```python
from build123d import *

# Parameters (mm, degrees)
SKETCH1_R               = 21
SKETCH1_R_2             = 17
BOSS_EXTRUDE1_DEPTH     = 6
SKETCH2_W               = 42
SKETCH2_H               = 3
CUT_EXTRUDE1_DEPTH      = 25.812
SKETCH3_W               = 34
SKETCH3_H               = 6
SKETCH3_W_2             = 33.201655863
SKETCH3_H_2             = 2.84
BOSS_EXTRUDE2_DEPTH     = 5.334
CUT_EXTRUDE2_START      = -19.05
SKETCH4_R               = 24.04163056
SKETCH4_R_2             = 21
CUT_EXTRUDE2_DEPTH      = 19.05
SKETCH5_R               = 1.4
CUT_EXTRUDE3_DEPTH      = 19.05
CHAMFER1_SIZE           = 1.279400032
CHAMFER2_SIZE           = 1.279400032
FILLET2_R               = 1.27
SKETCH8_R               = 0.85
CUT_EXTRUDE7_DEPTH      = 15.494
FILLET3_R               = 1.27
CUT_EXTRUDE8_DEPTH      = 19.812
CUT_EXTRUDE8_DEPTH_BACK = 28.194
SKETCH9_R               = 0.875


with BuildPart() as part:
    # Sketch1 → Boss-Extrude1 (new body)
    with BuildSketch(Plane(origin=(0, 0, 0), x_dir=(1, 0, 0), z_dir=(0, 1, 0))):
        with Locations(Location((0, 0, 0), (0, 0, 270))):
            Circle(SKETCH1_R)
        with Locations(Location((0, 0, 0), (0, 0, 270))):
            Circle(SKETCH1_R_2, mode=Mode.SUBTRACT)
    extrude(amount=BOSS_EXTRUDE1_DEPTH)

    # Sketch2 → Cut-Extrude1 (cut)
    with BuildSketch(Plane(origin=(0, 0, 0), x_dir=(0, 0, -1), z_dir=(1, 0, 0))):
        with Locations((0, 3)):
            Rectangle(SKETCH2_W, SKETCH2_H)
    extrude(amount=-CUT_EXTRUDE1_DEPTH, mode=Mode.SUBTRACT)

    # Sketch3 → Boss-Extrude2 (add)
    with BuildSketch(Plane.ZY.offset(-17)):
        with Locations((0, 3)):
            Rectangle(SKETCH3_W, SKETCH3_H)
        with Locations((0.110091931, 2.900051081)):
            Rectangle(SKETCH3_W_2, SKETCH3_H_2, mode=Mode.SUBTRACT)
    extrude(amount=BOSS_EXTRUDE2_DEPTH)

    # Sketch4 → Cut-Extrude2 (cut)
    with BuildSketch(Plane(origin=(0, 6, 0), x_dir=(1, 0, 0), z_dir=(0, 1, 0)).offset(CUT_EXTRUDE2_START)):
        Circle(SKETCH4_R)
        with Locations(Location((0, 0, 0), (0, 0, 270))):
            Circle(SKETCH4_R_2, mode=Mode.SUBTRACT)
    extrude(amount=CUT_EXTRUDE2_DEPTH, mode=Mode.SUBTRACT)

    # Sketch5 → Cut-Extrude3 (cut)
    with BuildSketch(Plane(origin=(21, 0, 0), x_dir=(0, 0, -1), z_dir=(1, 0, 0))):
        with Locations((0, 3)):
            Circle(SKETCH5_R)
    extrude(amount=-CUT_EXTRUDE3_DEPTH, mode=Mode.SUBTRACT)

    # Chamfer1
    chamfer1_edges = [part.edges().sort_by_distance(p)[0] for p in [
        (11.666, 6, 0),
        (11.666, 0, 0),
    ]]
    chamfer(chamfer1_edges, length=CHAMFER1_SIZE)

    # Chamfer2
    chamfer2_edges = [part.edges().sort_by_distance(p)[0] for p in [
        (-15.432460197, 0, -7.130159344),
        (-15.432460197, 6, -7.130159344),
    ]]
    chamfer(chamfer2_edges, length=CHAMFER2_SIZE)

    # Fillet2
    fillet2_edges = [part.edges().sort_by_distance(p)[0] for p in [
        (-12.328828006, 6, -17),
        (-12.328828006, 0, -17),
    ]]
    fillet(fillet2_edges, radius=FILLET2_R)

    # Sketch8 → Cut-Extrude7 (cut)
    with BuildSketch(Plane(origin=(0, 6, 0), x_dir=(1, 0, 0), z_dir=(0, 1, 0))):
        with Locations(Location((-18.993118417, 0, 0), (0, 0, 327.808132049))):
            Circle(SKETCH8_R)
    extrude(amount=-CUT_EXTRUDE7_DEPTH, mode=Mode.SUBTRACT)

    # Fillet3
    fillet3_edges = [part.edges().sort_by_distance(p)[0] for p in [
        (12.305140757, 0.640259275, 12.638148503),
        (12.305140757, 0.640259275, -12.638148503),
        (12.305140757, 5.359740725, 12.638148503),
        (12.305140757, 5.359740725, -12.638148503),
    ]]
    fillet(fillet3_edges, radius=FILLET3_R)

    # Sketch9 → Cut-Extrude8 (cut, two sides: drawn at the far end of the back side and taken through both)
    with BuildSketch(Plane.XY.offset(-CUT_EXTRUDE8_DEPTH_BACK)):
        with Locations(Location((14.157633808, 3, 0), (0, 0, 180))):
            Circle(SKETCH9_R)
    extrude(amount=CUT_EXTRUDE8_DEPTH + CUT_EXTRUDE8_DEPTH_BACK, mode=Mode.SUBTRACT)


solid = part.part
```
Part model, mm, in its own coordinate system. A direction names the side the tool comes from. Round coordinates to 2 decimals unless told otherwise and drop trailing zeros. Write each loop counter-clockwise with the first axis right and the second up, starting at its lowest first coordinate (ties: lowest second). Pieces come first, ordered by that corner, then holes.
Item 1: Cut at A-A, the plane y = 3. Give the cut face in (x, z), plus the area to 3 significant figures.
Results:
outline: (0, -21) arc R21 ccw to (13.28, -16.27) - (13.28, -10.61) arc R17 cw to (0, -17) - close; (0, 17) arc R17 cw to (13.28, 10.61) - (13.28, 16.27) arc R21 ccw to (0, 21) - close; (15.03, -14.66) arc R21 ccw to (20.95, -1.4) - (16.94, -1.4) arc R17 cw to (15.03, -7.94) - close; (15.03, 7.94) arc R17 cw to (16.94, 1.4) - (20.95, 1.4) arc R21 ccw to (15.03, 14.66) - close
area: 206 mm2
Item 2: Probe L1, parallel to X at y = 5.45, z = 0; L2, parallel to Y at x = -9.5, z = -16; L3, parallel to Y at x = 17.25, z = 0. List the from-to ranges inside material, lowest first.
Results:
L1: x = -20.78 to -19.84, -18.14 to -17.73, 12.4 to 20.78
L2: y = 0 to 1.5, 4.5 to 6
L3: y = 0 to 1.6, 4.4 to 6
Item 3: Drop flat-ended pins along their axis: pin 1 Ø1.5 at (x, y) = (6, 1) entering from -Z; pin 2 Ø8 at (x, z) = (-14, 2) entering from +Y; pin 3 Ø2.5 at (x, y) = (14.16, 3) entering from +Z; pin 4 Ø23 at (x, z) = (-8, 7.5) entering from -Y. Give the stop position or say it passes through.
Results:
pin 1: stops at z = -20.32
pin 2: stops at y = 5.86
pin 3: stops at z = 16.56
pin 4: stops at y = 0
Item 4: Which spindle directions (+Z, -Z, +X, -X, +Y, -Y) get a long thin tool onto all of the face, cutting with end or side? Do faces 5 (the flat face through (12.315, 0.631, -0.175)), 6 (the flat face through (0, 3, -19)). Say none if no direction does.
Results:
face 5: -Y
face 6: +Z, -Z, -X
Item 5: Two-plate mould, pull along Z, no slides. Class faces 1 (the flat face through (-17.5, 1.5, 0.1)), 2 (the flat face through (12.315, 5.369, -0.175)), 3 (the flat face through (14, 4.32, 5)), 4 (the cylindrical face through (20.82, 2.98, -2.73)): +Z half, -Z half, draft (parallel to the pull), parting line (faces both ways), or undercut.
Results:
face 1: draft
face 2: undercut
face 3: undercut
face 4: parting line
Item 6: Cut at B-B, the plane x = -6.5. Count the separate pieces of the cut face and the enclosed holes in it, plus the area to 3 significant figures.
Results:
separate pieces: 4
enclosed holes: 0
area: 20.6 mm2
